Autodesk Inventor part; units mm, degrees
ref_plane "YZ Plane" through (0, 0, 0) normal (1, 0, 0) x (0, 1, 0)
ref_plane "XZ Plane" through (0, 0, 0) normal (0, 1, 0) x (-1, 0, 0)
ref_plane "XY Plane" through (0, 0, 0) normal (0, 0, 1) x (1, 0, 0)
sketch "Sketch1" plane through (0, 0, 0) normal (0, 1, 0) x (-1, 0, 0)
  line L0 (3.2, 1.8475) -> (3.2, -1.8475)
  line L1 (3.2, -1.8475) -> (0, -3.695)
  line L2 (0, -3.695) -> (-3.2, -1.8475)
  line L3 (-3.2, -1.8475) -> (-3.2, 1.8475)
  line L4 (-3.2, 1.8475) -> (0, 3.695)
  line L5 (0, 3.695) -> (3.2, 1.8475)
  point P0 (0, 0)
  point P1 (3.2, 0)
  point P2 (-3.2, 0)
  dimension "d0" = 6.4
  dimension "d1" = 120
  dimension "d2" = 6.4
extrude "Extrusion1" add sketch "Sketch1" along normal blind 15.2
sketch "Sketch3" plane through (0, 0, 0) normal (0, -1, 0) x (1, 0, 0)
  circle A0 centre (0, 0) radius 1.4224
  dimension "d8" = 2.8448
extrude "Extrusion3" cut sketch "Sketch3" against normal blind 6.4
sketch "Sketch4" plane through (0, 15.2, 0) normal (0, 1, 0) x (1, 0, 0)
  circle A0 centre (0, 0) radius 1.4224
extrude "Extrusion4" add sketch "Sketch4" along normal blind 4.75
properties part number "pc104standoff" material "Stainless Steel"
Design review of the part built by this model. Coordinates are the model's own, in mm. A direction names the side the tool comes from. Coordinates: 2 decimals unless noted, no trailing zeros. Write each loop counter-clockwise with the first axis right and the second up, starting at its lowest first coordinate (ties: lowest second). Pieces come first, ordered by that corner, then holes. Notation, with made-up numbers: M 35,71.25 L 53,71.25 A16 cw 53,92.25 Z; hole C 21.5,77 d10. An arc over 180 degrees is marked long. Answer as a JSON object with one key per item and string values.
Item 1: Wall thickness on probe 1 along Y at (x, z) = (-0.5, 1); probe 2 along Y at (x, z) = (-1.25, 1.25); probe 3 along X at (y, z) = (3.5, 1): over which ranges is each line inside the solid? List them lowest first.
Outcome:
{"probe 1": "6.4 to 19.95", "probe 2": "0 to 15.2", "probe 3": "-3.2 to -1.01, 1.01 to 3.2"}
Item 2: Add section C-C, the plane y = 11.25. Give the boundary of the cut face in (x, z) (1 decimal), and give its area (3 significant figures).
Outcome:
{"outline": "M -3.2,-1.8 L 0,-3.7 L 3.2,-1.8 L 3.2,1.8 L 0,3.7 L -3.2,1.8 Z", "area": "35.5 mm²"}
Item 3: Draft analysis for pull direction Z (two halves, no side actions). For faces 3 (the cylindrical face through (-0.31, 3.16, -1.39)), 4 (the flat face through (0, 0, -2)), 5 (the flat face through (0, 6.4, 0)), 6 (the flat face through (-1.62, 7.49, -2.76)), state which applies: pulls with the +Z half, pulls with the -Z half, needs draft (parallel to the pull), parting line crosses it, or undercut.
Outcome:
{"face 3": "undercut", "face 4": "needs draft", "face 5": "undercut", "face 6": "pulls with the -Z half"}
Item 4: Insertion check: pin 1 Ø2.5 at (x, z) = (0, 0) entering from -Y; pin 2 Ø3 at (x, z) = (-2.5, -1) entering from +Y. Each pin has a flat end and moves straight along its axis. Give the tip position at first contact, or say it passes through.
Outcome:
{"pin 1": "y = 6.4", "pin 2": "y = 19.95"}
Item 5: Add section D-D, the plane x = -0.75. Give the boundary of the cut face in (y, z).
Outcome:
{"outline": "M 0,-3.26 L 15.2,-3.26 L 15.2,-1.21 L 19.95,-1.21 L 19.95,1.21 L 15.2,1.21 L 15.2,3.26 L 0,3.26 L 0,1.21 L 6.4,1.21 L 6.4,-1.21 L 0,-1.21 Z"}
Item 6: Machinability: for faces 1 (the flat face through (0, 15.2, -2)), 2 (the flat face through (-3.2, 7, 0)), which of the approach directions +Z, -Z, +X, -X, +Y, -Y give a long, thin tool a straight path to every point of the face, cutting with its end or side? Answer none if there is none.
Outcome:
{"face 1": "+Y", "face 2": "+Z, -Z, -X, +Y, -Y"}
Item 7: Add section B-B, the plane z = 0. Give the boundary of the cut face in (x, y), and give its area (3 significant figures).
Outcome:
{"outline": "M -3.2,0 L -1.42,0 L -1.42,6.4 L 1.42,6.4 L 1.42,0 L 3.2,0 L 3.2,15.2 L 1.42,15.2 L 1.42,19.95 L -1.42,19.95 L -1.42,15.2 L -3.2,15.2 Z", "area": "92.6 mm²"}
Item 8: Add section A-A, the plane y = 6. Give the boundary of the cut face in (x, z) (1 decimal), and give its area (3 significant figures).
Outcome:
{"outline": "M -3.2,-1.8 L 0,-3.7 L 3.2,-1.8 L 3.2,1.8 L 0,3.7 L -3.2,1.8 Z; hole C 0,0 d2.8", "area": "29.1 mm²"}
